CAD build for the part. Positions are in the model's coordinates, mm. Face numbers are marked on the shaded views. Coordinates: 2 decimals unless noted, no trailing zeros. Write item = value, one per line.
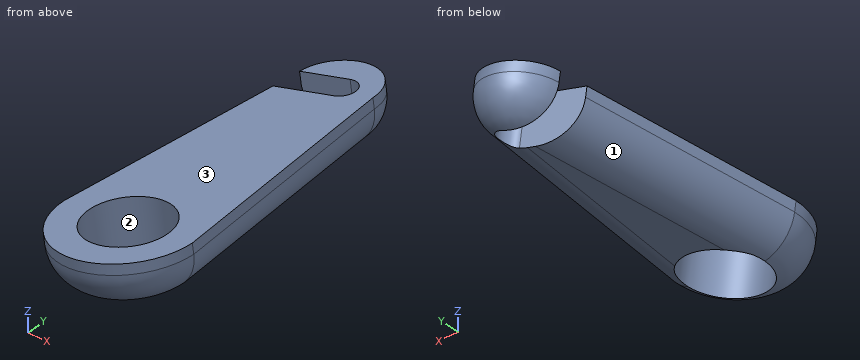
from build123d import *

# Parameters (mm, degrees)
BASE_EXTRUDE_DEPTH = 6.35
FILLET1_R          = 5
CUT_EXTRUDE1_START = -6.35
CUT_EXTRUDE1_DEPTH = 6.350746
SKETCH4_R          = 5.334
CUT_EXTRUDE2_DEPTH = 6.35


with BuildPart() as part:
    # Sketch1 → Base Extrude (new body)
    with BuildSketch(Plane(origin=(8.114628625, -3.283425705, -55.67660861), x_dir=(-0.989545354, 0, -0.144222022), z_dir=(0.144222022, 0, -0.989545354))):
        with BuildLine():
            Line((-1.106091457, 205.484448373), (2.665349365, 238.484448373))
            ThreePointArc((2.665349365, 238.484448373), (7.915349365, 243.734448373), (13.165349365, 238.484448373))
            Line((13.165349365, 238.484448373), (16.673908543, 205.484448373))
            ThreePointArc((16.673908543, 205.484448373), (7.783908543, 196.594448373), (-1.106091457, 205.484448373))
        make_face()
    extrude(amount=BASE_EXTRUDE_DEPTH)

    # Fillet1
    fillet1_edges = [part.edges().sort_by_distance(p)[0] for p in [
        (-5.733211058, 218.701022668, -64.111960662),
        (1.327907925, 193.311022668, -63.082832637),
        (8.258960253, 218.701022668, -62.072661274),
        (1.19784127, 240.451022668, -63.101789298),
    ]]
    fillet(fillet1_edges, radius=FILLET1_R)

    # Sketch3 → Cut-Extrude1 (cut)
    with BuildSketch(Plane(origin=(9.030438463, -3.283425705, -61.96022161), x_dir=(-0.989545354, 0, -0.144222022), z_dir=(0.144222022, 0, -0.989545354)).offset(CUT_EXTRUDE1_START)):
        with BuildLine():
            Line((14.3026167, 234.886394841), (6.516843813, 236.725345777))
            ThreePointArc((6.516843813, 236.725345777), (5.178808874, 238.890908637), (7.344371734, 240.228943576))
            Line((7.344371734, 240.228943576), (15.130144622, 238.38999264))
            ThreePointArc((15.130144622, 238.38999264), (16.468179561, 236.22442978), (14.3026167, 234.886394841))
        make_face()
    extrude(amount=CUT_EXTRUDE1_DEPTH, mode=Mode.SUBTRACT)


with BuildPart() as body_2:
    # Mirror2: mirrored copy
    add(part.part.mirror(Plane(origin=(-103.213448145, 0, -15.042920567), x_dir=(-0.144222022, 0, 0.989545354), z_dir=(0.989545354, 0, 0.144222022))))


with BuildPart() as part_1:
    add(part.part)

    # Sketch4 → Cut-Extrude2 (cut)
    with BuildSketch(Plane(origin=(9.030438463, 0, -61.96022161), x_dir=(-0.989545354, 0, -0.144222022), z_dir=(0.144222022, 0, -0.989545354))):
        with Locations((7.783908543, 202.201022668)):
            Circle(SKETCH4_R)
    cut_extrude2 = extrude(amount=-CUT_EXTRUDE2_DEPTH, mode=Mode.SUBTRACT)


with BuildPart() as body_2_1:
    add(body_2.part)

    # Mirror3: Cut-Extrude2 across plane
    add(cut_extrude2.mirror(Plane(origin=(-103.213448145, 0, -15.042920567), x_dir=(-0.144222022, 0, 0.989545354), z_dir=(0.989545354, 0, 0.144222022))), mode=Mode.SUBTRACT)


solid = part_1.part
(1) Pin check, flat tips, straight feed: pin 1 Ø1 at (x, z) = (0, -59) entering from -Y; pin 2 Ø4 at (y, z) = (210.5, -60.5) entering from +X; pin 3 Ø1 at (x, y) = (2.5, 208) entering from -Z. Stop position of each tip, or through.
Evaluation:
pin_1 = 193.33
pin_2 = 8.51
pin_3 = -62.98
(2) Wall check: line 1 (Y direction, x = 1.25, z = -59.5); line 2 (Y direction, x = -0.25, z = -62.25); line 3 (X direction, y = 203.5, z = -60.5). Give the ranges that are in metal, low to high. Write a range as from..to.
Evaluation:
line_1 = 193.54..196.89, 207.52..233.25, 236.95..240.21
line_2 = 195.39..197.07, 207.34..232.8, 236.5..238.25
line_3 = -7.76..-4.28, 6.18..8.37
(3) Slice it at A-A, the plane x = -2.5. State how many separate pieces and enclosed holes the cut face has, then the cut area to 3 significant figures.
Evaluation:
separate_pieces = 3
enclosed_holes = 0
area = 191 mm²
(4) Pull direction Y, two halves, no side cores. Call the marked faces 1, 2 and 3: +Y half, -Y half, draft (parallel to the pull), parting line (faces both ways), or undercut.
Evaluation:
face_1 = +Y half
face_2 = undercut
face_3 = draft
